Check sheet for the modelled part. Datum: model origin and axes. Units: mm. Coordinates: 2 decimals unless noted, no trailing zeros. Loops run counter-clockwise (first coordinate to the right, second up) from the corner with the lowest first, then second, coordinate; pieces in that order, holes last.
```python
from build123d import *

# Parameters (mm, degrees)
F0_W     = 815
F0_H     = 1975
F0_W_2   = 610
F0_H_2   = 392.25
F1_DEPTH = 22.5
F2_SIZE2 = 17
F2_SIZE  = 6
F3_SIZE2 = 13
F3_SIZE  = 6


with BuildPart() as f1:
    # F0 (on Front) → F1 (new body, symmetric)
    with BuildSketch(Plane.XZ):
        Rectangle(F0_W, F0_H)
        with Locations((0, -551.375)):
            Rectangle(F0_W_2, F0_H_2, mode=Mode.SUBTRACT)
        with Locations((0, -137.125)):
            Rectangle(F0_W_2, F0_H_2, mode=Mode.SUBTRACT)
        with Locations((0, 277.125)):
            Rectangle(F0_W_2, F0_H_2, mode=Mode.SUBTRACT)
        with Locations((0, 691.375)):
            Rectangle(F0_W_2, F0_H_2, mode=Mode.SUBTRACT)
    extrude(amount=F1_DEPTH, both=True)

    # F2
    f2_edges = [f1.edges().sort_by_distance(p)[0] for p in [
        (305, -22.5, -551.375),
        (0, -22.5, -355.25),
        (305, -22.5, -137.125),
        (0, -22.5, 59),
        (305, -22.5, 277.125),
        (0, -22.5, 473.25),
        (305, -22.5, 691.375),
        (0, -22.5, 887.5),
        (-305, -22.5, 691.375),
        (0, -22.5, 495.25),
        (-305, -22.5, 277.125),
        (0, -22.5, 81),
        (-305, -22.5, -137.125),
        (0, -22.5, -333.25),
        (-305, -22.5, -551.375),
        (0, -22.5, -747.5),
    ]]
    f2_side = f1.faces().sort_by_distance((0, -22.5, 966.13449))[0]
    chamfer(f2_edges, length=F2_SIZE, length2=F2_SIZE2, reference=f2_side)

    # F3
    f3_edges = [f1.edges().sort_by_distance(p)[0] for p in [
        (0, 22.5, -747.5),
        (305, 22.5, -551.375),
        (0, 22.5, -355.25),
        (-305, 22.5, -551.375),
        (-305, 22.5, -137.125),
        (0, 22.5, 59),
        (-305, 22.5, 277.125),
        (0, 22.5, -333.25),
        (305, 22.5, -137.125),
        (0, 22.5, 81),
        (305, 22.5, 277.125),
        (0, 22.5, 473.25),
        (305, 22.5, 691.375),
        (0, 22.5, 887.5),
        (-305, 22.5, 691.375),
        (0, 22.5, 495.25),
    ]]
    f3_side = f1.faces().sort_by_distance((0, 22.5, 966.13449))[0]
    chamfer(f3_edges, length=F3_SIZE, length2=F3_SIZE2, reference=f3_side)


solid = f1.part
```
1) Section check A-A on z = -642. Enter the section's corners in (x, y), plus the area to 4 significant figures.
Answer sheet:
outline: (-407.5, -22.5) - (-311, -22.5) - (-305, -5.5) - (-305, 9.5) - (-311, 22.5) - (-407.5, 22.5) - close; (305, -5.5) - (311, -22.5) - (407.5, -22.5) - (407.5, 22.5) - (311, 22.5) - (305, 9.5) - close
area: 9,045 mm2
2) Scan lines: line 1 (Z direction, x = 140, y = 2); line 2 (X direction, y = 9, z = 514); line 3 (Z direction, x = 45.5, y = 13.5). Record each from-to range of solid material in increasing order.
Answer sheet:
line 1: z = -987.5 to -747.5, -355.25 to -333.25, 59 to 81, 473.25 to 495.25, 887.5 to 987.5
line 2: x = -407.5 to -305, 305 to 407.5
line 3: z = -987.5 to -749.35, -353.4 to -335.1, 60.85 to 79.15, 475.1 to 493.4, 889.35 to 987.5
3) Section check C-C on y = -15. Enter the section's corners in (x, z), plus the area to 3 significant figures.
Answer sheet:
outline: (-407.5, -987.5) - (407.5, -987.5) - (407.5, 987.5) - (-407.5, 987.5) - close; hole (-308.35, -750.85) - (308.35, -750.85) - (308.35, -351.9) - (-308.35, -351.9) - close; hole (-308.35, -336.6) - (308.35, -336.6) - (308.35, 62.35) - (-308.35, 62.35) - close; hole (-308.35, 77.65) - (308.35, 77.65) - (308.35, 476.6) - (-308.35, 476.6) - close; hole (-308.35, 491.9) - (308.35, 491.9) - (308.35, 890.85) - (-308.35, 890.85) - close
area: 625,000 mm2
4) Section check B-B on x = 240. Give the number of separate pieces and of enclosed holes in the cut face, plus the area to 4 significant figures.
Answer sheet:
separate pieces: 5
enclosed holes: 0
area: 17,550 mm2
